Input: part model. Units: mm. Frame: model coordinates. A direction names the side the tool comes from. Give positions to 0.01 mm unless a question says otherwise; leave off trailing zeros. Loops run counter-clockwise (first coordinate to the right, second up) from the corner with the lowest first, then second, coordinate; pieces in that order, holes last. Notation, with made-up numbers: M 51,89 L 98,89 A33 ccw 98,124 Z; hole C 28.5,29.25 d9. An arc over 180 degrees is marked long. Answer as a JSON object with one key per item and string values. Group by question number.
1) First-contact query: P1, Ø0.5, axis at y = -4, z = 0.5, coming from the -X side; P2, Ø0.7, axis at y = -5, z = -1.5, coming from the -X side; P3, Ø1.6, axis at y = -4, z = 1.5, coming from the +X side. Flat tips, straight axial feed; report the tip coordinate or a pass-through.
2) Section query B-B on y = -4. Return loops of the section in (x, z) (3 decimals), plus the area to 3 significant figures.
3) Section query D-D on z = 3.25. Return loops of the section in (x, y).
4) Access query for faces 4 (the flat face through (2, -7.8, -2)), 5 (the flat face through (2, -4, -0.89)). Directions: +Z, -Z, +X, -X, +Y, -Y. A direction counts if a zero-diameter tool reaches every point of the face in a straight line with its end or side. Return the directions, or none.
5) Section query C-C on z = -2. Return loops of the section in (x, y).
6) Section query A-A on x = 0. Return loops of the section in (y, z) (3 decimals).
7) Ray query, L1, parallel to X at y = -3.25, z = -1; L2, parallel to Z at x = 2.25, y = -1.75. Return the intervals inside material, ascending.
8) Draft query along Z for faces 1 (the flat face through (2, -4, 0.89)), 2 (the cylindrical face through (-0.797, -3.845, -3.588)), 3 (the flat face through (2, 0, -2)). Return one class per face: +Z half, -Z half, draft (parallel to the pull), parting line (faces both ways), or undercut.
from build123d import *

# Parameters (mm, degrees)
F0_R     = 3.675
F1_DEPTH = 7.8
F2_DEPTH = 7.8


# Not quite as in the source:
# - a feature names something its author has since deleted; it is built from what else it names


with BuildPart() as f1:
    # F0 (on Front) → F1 (new body)
    with BuildSketch(Plane.XZ):
        Circle(F0_R)
        with BuildLine():
            Line((-2.375, 0.2181742423), (-2.375, 0.89))
            Line((-2.375, 0.89), (-2.2127189157, 0.89))
            ThreePointArc((-2.2127189157, 0.89), (-1.6864496731, 1.6864496731), (-0.89, 2.2127189157))
            Line((-0.89, 2.2127189157), (-0.89, 2.375))
            Line((-0.89, 2.375), (-0.2181742423, 2.375))
            ThreePointArc((-0.2181742423, 2.375), (0, 2.385), (0.2181742423, 2.375))
            Line((0.2181742423, 2.375), (0.89, 2.375))
            Line((0.89, 2.375), (0.89, 2.2127189157))
            ThreePointArc((0.89, 2.2127189157), (1.6864496731, 1.6864496731), (2.2127189157, 0.89))
            Line((2.2127189157, 0.89), (2.375, 0.89))
            Line((2.375, 0.89), (2.375, 0.2181742423))
            ThreePointArc((2.375, 0.2181742423), (2.3824986884, 0.1092016483), (2.385, 0))
            ThreePointArc((2.385, 0), (2.3824986884, -0.1092016483), (2.375, -0.2181742423))
            Line((2.375, -0.2181742423), (2.375, -0.89))
            Line((2.375, -0.89), (2.2127189157, -0.89))
            ThreePointArc((2.2127189157, -0.89), (1.6864496731, -1.6864496731), (0.89, -2.2127189157))
            Line((0.89, -2.2127189157), (0.89, -2.375))
            Line((0.89, -2.375), (0.2181742423, -2.375))
            ThreePointArc((0.2181742423, -2.375), (0, -2.385), (-0.2181742423, -2.375))
            Line((-0.2181742423, -2.375), (-0.89, -2.375))
            Line((-0.89, -2.375), (-0.89, -2.2127189157))
            ThreePointArc((-0.89, -2.2127189157), (-1.6864496731, -1.6864496731), (-2.2127189157, -0.89))
            Line((-2.2127189157, -0.89), (-2.375, -0.89))
            Line((-2.375, -0.89), (-2.375, -0.2181742423))
            ThreePointArc((-2.375, -0.2181742423), (-2.385, 0), (-2.375, 0.2181742423))
        make_face(mode=Mode.SUBTRACT)
    extrude(amount=F1_DEPTH)

    # F0 (on Front) → F2 (join)
    with BuildSketch(Plane.XZ):
        with BuildLine():
            ThreePointArc((-0.89, 2.2127189157), (-1.6864496731, 1.6864496731), (-2.2127189157, 0.89))
            Line((-2.2127189157, 0.89), (-0.89, 0.89))
            Line((-0.89, 0.89), (-0.89, 2.2127189157))
        make_face()
        with BuildLine():
            Line((0.89, 2.2127189157), (0.89, 0.89))
            Line((0.89, 0.89), (2.2127189157, 0.89))
            ThreePointArc((2.2127189157, 0.89), (1.6864496731, 1.6864496731), (0.89, 2.2127189157))
        make_face()
        with BuildLine():
            Line((-0.89, -0.89), (-2.2127189157, -0.89))
            ThreePointArc((-2.2127189157, -0.89), (-1.6864496731, -1.6864496731), (-0.89, -2.2127189157))
            Line((-0.89, -2.2127189157), (-0.89, -0.89))
        make_face()
        with BuildLine():
            Line((2.2127189157, -0.89), (0.89, -0.89))
            Line((0.89, -0.89), (0.89, -2.2127189157))
            ThreePointArc((0.89, -2.2127189157), (1.6864496731, -1.6864496731), (2.2127189157, -0.89))
        make_face()
    extrude(amount=F2_DEPTH)


solid = f1.part
Output:
{
 "1": {"P1": "stops at x = -3.67", "P2": "stops at x = -3.49", "P3": "stops at x = 3.61"},
 "2": {"outline": "C 0,0 d7.35; hole M -2.375,-0.89 L -0.89,-0.89 L -0.89,-2.375 L -0.218,-2.375 A2.385 ccw 0.218,-2.375 L 0.89,-2.375 L 0.89,-0.89 L 2.375,-0.89 L 2.375,-0.218 A2.385 ccw 2.375,0.218 L 2.375,0.89 L 0.89,0.89 L 0.89,2.375 L 0.218,2.375 A2.385 ccw -0.218,2.375 L -0.89,2.375 L -0.89,0.89 L -2.375,0.89 L -2.375,0.218 A2.385 ccw -2.375,-0.218 Z", "area": "28.7 mm^2"},
 "3": {"outline": "M -1.72,-7.8 L 1.72,-7.8 L 1.72,0 L -1.72,0 Z"},
 "4": {"face 4": "+Z, -Z, +X, -X, -Y", "face 5": "+Y, -Y"},
 "5": {"outline": "M -3.08,-7.8 L -0.89,-7.8 L -0.89,0 L -3.08,0 Z; M 0.89,-7.8 L 3.08,-7.8 L 3.08,0 L 0.89,0 Z"},
 "6": {"outline": "M -7.8,-3.675 L 0,-3.675 L 0,-2.385 L -7.8,-2.385 Z; M -7.8,2.385 L 0,2.385 L 0,3.675 L -7.8,3.675 Z"},
 "7": {"L1": "x = -3.54 to -0.89, 0.89 to 3.54", "L2": "z = -2.91 to -0.89, 0.89 to 2.91"},
 "8": {"face 1": "undercut", "face 2": "parting line", "face 3": "draft"}
}
